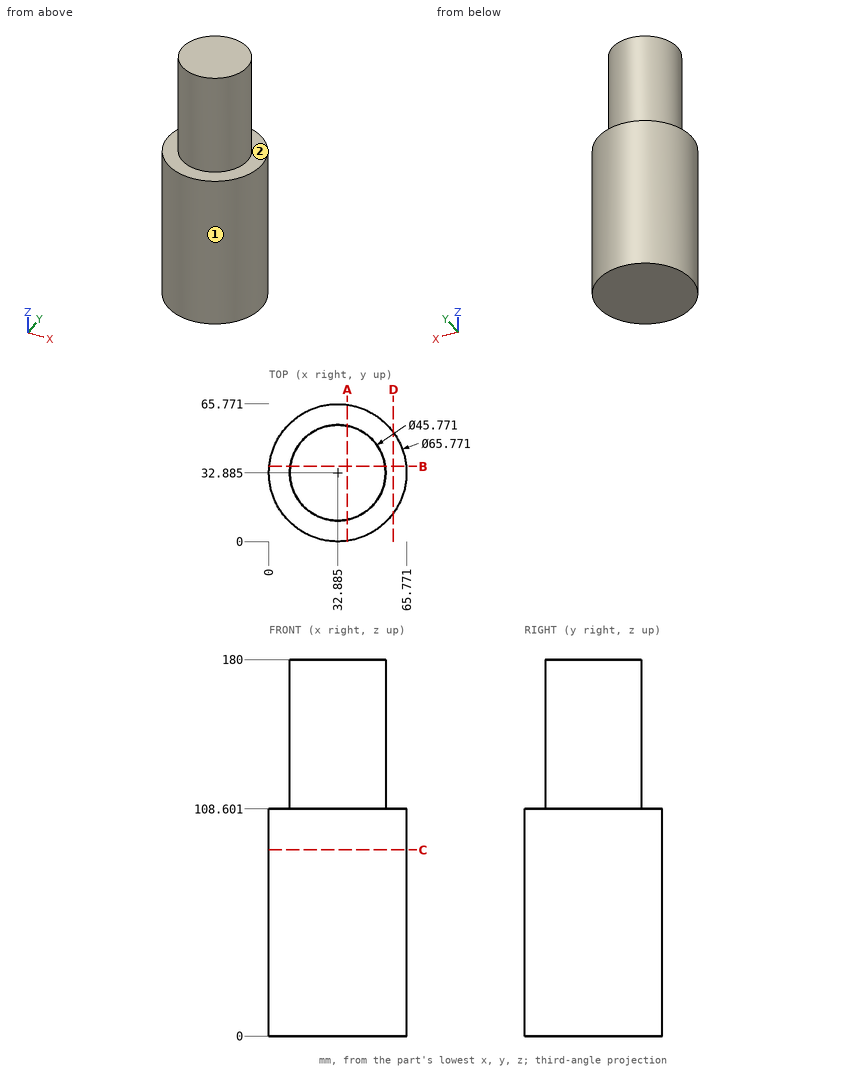
The figure shows three views and two pictorial views of one solid part (mm, origin at its lowest corner). Answer the questions. A direction names the side the tool comes from. Give positions to 0.01 mm unless a question says otherwise; leave off trailing zeros. Loops run counter-clockwise (first coordinate to the right, second up) from the corner with the lowest first, then second, coordinate; pieces in that order, holes last. Notation, with made-up numbers: M -35.75,73.25 L 8.25,73.25 A15 ccw 8.25,88.25 Z; hole C -36,-26 d6. An arc over 180 degrees is marked long. Write each question's results on one line, items separated by ' | '.
1. Section A-A on x = 37.5 is taken. Give the vertices of the cut face in (y, z) (1 decimal).
Values:
outline: M 0.3,0 L 65.4,0 L 65.4,108.6 L 55.3,108.6 L 55.3,180 L 10.5,180 L 10.5,108.6 L 0.3,108.6 Z
2. Section B-B on y = 36 is taken. Give the vertices of the cut face in (x, z).
Values:
outline: M 0.15,0 L 65.62,0 L 65.62,108.6 L 55.56,108.6 L 55.56,180 L 10.21,180 L 10.21,108.6 L 0.15,108.6 Z
3. Section D-D on x = 59.5 is taken. Give the vertices of the cut face in (y, z).
Values:
outline: M 13.57,0 L 52.2,0 L 52.2,108.6 L 13.57,108.6 Z
4. A tool of negligible diameter and unlimited length cuts with its end or side. For the marked faces 1 and 2, from which of +Z, -Z, +X, -X, +Y, -Y can it reach the whole face along a straight path? Write none if from no direction.
Values:
face 1: +Z, -Z | face 2: +Z
5. Straight lines are drawn through the part: line 1 (Z direction, x = 19.5, y = 60.5); line 2 (X direction, y = 52, z = 67) (1 decimal); line 3 (X direction, y = 12.5, z = 35.5). For each, find the intervals that lie inside material, in ascending order. Write a range as [from, to].
Values:
line 1: z = [0, 108.6] | line 2: x = [6.1, 59.6] | line 3: x = [7.08, 58.69]
6. Given pin 1 (4 mm diameter, centred on y = 24, z = 75, fed in from -X); pin 2 (8 mm diameter, centred on y = 45, z = 63, fed in from -X); pin 3 (12 mm diameter, centred on y = 34.5, z = 151.5, fed in from -X), each flat-ended and moving along its own axis, determine where each tip first touches the part or whether it passes through.
Values:
pin 1: stops at x = 0.73 | pin 2: stops at x = 1.02 | pin 3: stops at x = 10
7. Section C-C on z = 89 is taken. Give the vertices of the cut face in (x, y) (1 decimal).
Values:
outline: C 32.9,32.9 d65.8
